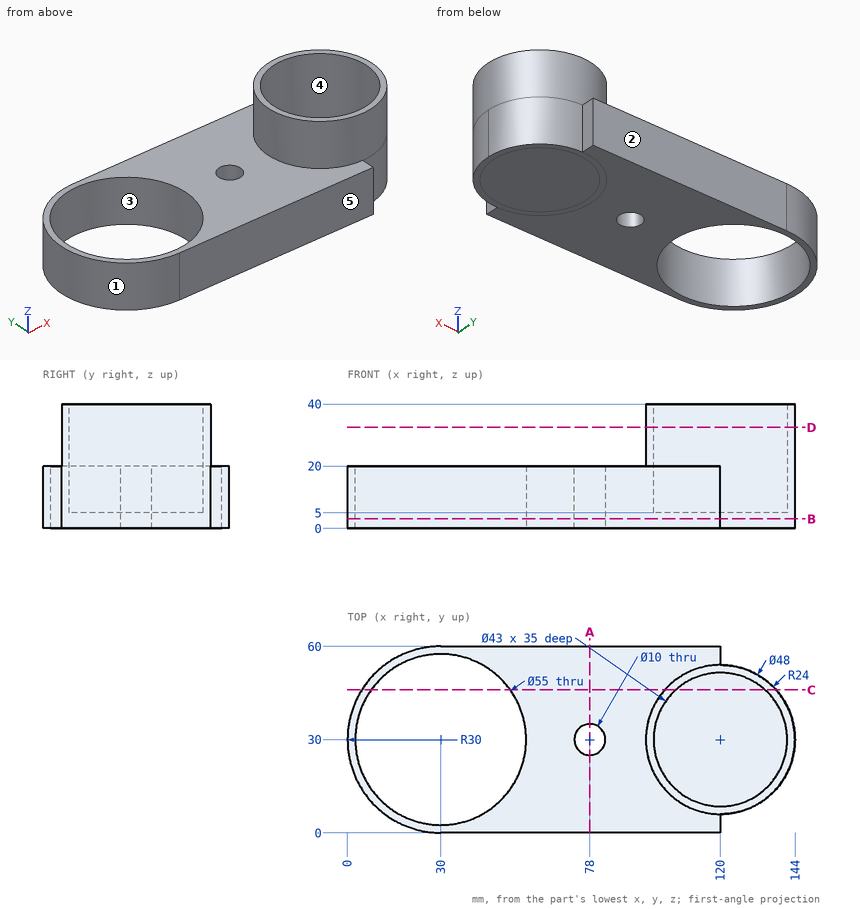
Input: dimensioned drawing with shaded views. Units: mm. Origin: part minimum x, y, z. A direction names the side the tool comes from. Coordinates: 2 decimals unless noted, no trailing zeros. Loops run counter-clockwise (first coordinate to the right, second up) from the corner with the lowest first, then second, coordinate; pieces in that order, holes last. Notation, with made-up numbers: (59.25, 77) - (97.25, 77) arc R21 cw to (97.25, 101) - close; hole circle Ø3 at (27.25, 36.5). An arc over 180 degrees is marked (long way). One line per question, with ' | ' between items. Start each with the question number.
(1) Cut plane D-D on z = 32.5. Output: boundary loops of the cut face in (x, y), and give its area (3 significant figures).
(2) Reachability of the marked faces 4 and 5 from +Z, -Z, +X, -X, +Y, -Y: full face, straight path, thin tool, end or side. Return the list, or none.
(3) Cut plane A-A on x = 78. Output: boundary loops of the cut face in (y, z), and give its area (3 significant figures).
(4) Cut plane C-C on y = 46. Output: boundary loops of the cut face in (x, z), and give its area (3 significant figures).
(5) Ray query, L1, parallel to X at y = 42, z = 18; L2, parallel to Y at x = 78, z = 12; L3, parallel to X at y = 37.5, z = 14. Return the intervals inside material, ascending. Write a range as from..to.
(6) Cut plane B-B on z = 3. Output: boundary loops of the cut face in (x, y).
(7) First-contact query: pin 1 (21.5 mm diameter, centred on x = 129.5, y = 34.5, fed in from +Z); pin 2 (1 mm diameter, centred on y = 8, z = 10.5, fed in from +X); pin 3 (1.5 mm diameter, centred on x = 83, z = 21.5, fed in from +Y); pin 4 (6.5 mm diameter, centred on y = 57.5, z = 9.5, fed in from +X). Flat tips, straight axial feed; report the tip coordinate or a pass-through.
(8) Draft query along X for the marked faces 1, 2 and 3. Return one class per face: +X half, -X half, draft (parallel to the pull), parting line (faces both ways), or undercut.
Here are the results:
1) outline: circle Ø48 at (120, 30); hole circle Ø43 at (120, 30) | area: 357 mm²
2) face 4: +Z | face 5: +Z, -Z, +X, -X, -Y
3) outline: (0, 0) - (25, 0) - (25, 20) - (0, 20) - close; (35, 0) - (60, 0) - (60, 20) - (35, 20) - close | area: 1,000 mm²
4) outline: (4.62, 0) - (7.63, 0) - (7.63, 20) - (4.62, 20) - close; (52.37, 0) - (137.89, 0) - (137.89, 40) - (134.36, 40) - (134.36, 5) - (105.64, 5) - (105.64, 40) - (102.11, 40) - (102.11, 20) - (52.37, 20) - close | area: 1,480 mm²
5) L1: 2.5..5.26, 54.74..102.16, 137.84..140.78 | L2: 0..25, 35..60 | L3: 0.95..3.54, 56.46..99.85, 140.15..142.8
6) outline: (30, 0) - (120, 0) - (120, 6) arc R24 ccw to (120, 54) - (120, 60) - (30, 60) arc R30 ccw to start; hole circle Ø55 at (30, 30); hole circle Ø10 at (78, 30)
7) pin 1: z = 5 | pin 2: x = 130.67 | pin 3: through | pin 4: x = 120
8) face 1: -X half | face 2: draft | face 3: undercut
